```python
from build123d import *

# Parameters (mm, degrees)
F0_R     = 1.5
F0_R_2   = 10
F1_DEPTH = 3
F2_R     = 5


with BuildPart() as f1:
    # F0 (on Top) → F1 (new body)
    with BuildSketch(Plane.XY):
        with BuildLine():
            Line((67.5, 27.96), (27.96, 67.5))
            Line((27.96, 67.5), (7.0710678119, 46.6110678119))
            ThreePointArc((7.0710678119, 46.6110678119), (0, 43.6821356237), (-7.0710678119, 46.6110678119))
            Line((-7.0710678119, 46.6110678119), (-27.96, 67.5))
            Line((-27.96, 67.5), (-67.5, 27.96))
            Line((-67.5, 27.96), (-46.6110678119, 7.0710678119))
            ThreePointArc((-46.6110678119, 7.0710678119), (-43.6821356237, 0), (-46.6110678119, -7.0710678119))
            Line((-46.6110678119, -7.0710678119), (-67.5, -27.96))
            Line((-67.5, -27.96), (-27.96, -67.5))
            Line((-27.96, -67.5), (-7.0710678119, -46.6110678119))
            ThreePointArc((-7.0710678119, -46.6110678119), (0, -43.6821356237), (7.0710678119, -46.6110678119))
            Line((7.0710678119, -46.6110678119), (27.96, -67.5))
            Line((27.96, -67.5), (67.5, -27.96))
            Line((67.5, -27.96), (46.6110678119, -7.0710678119))
            ThreePointArc((46.6110678119, -7.0710678119), (43.6821356237, 0), (46.6110678119, 7.0710678119))
            Line((46.6110678119, 7.0710678119), (67.5, 27.96))
        make_face()
        with Locations((9.5, -35.5)):
            Circle(F0_R, mode=Mode.SUBTRACT)
        with Locations((35.3553390593, -35.3553390593)):
            Circle(F0_R_2, mode=Mode.SUBTRACT)
        with Locations((0, -21.9203102168)):
            Circle(F0_R, mode=Mode.SUBTRACT)
        with Locations((35.5, -9.5)):
            Circle(F0_R, mode=Mode.SUBTRACT)
        with Locations((-35.5, 9.5)):
            Circle(F0_R, mode=Mode.SUBTRACT)
        with Locations((-21.9203102168, 0)):
            Circle(F0_R, mode=Mode.SUBTRACT)
        with Locations((-35.3553390593, 35.3553390593)):
            Circle(F0_R_2, mode=Mode.SUBTRACT)
        with Locations((-9.5, 35.5)):
            Circle(F0_R, mode=Mode.SUBTRACT)
        with Locations((21.9203102168, 0)):
            Circle(F0_R, mode=Mode.SUBTRACT)
        with Locations((0, 21.9203102168)):
            Circle(F0_R, mode=Mode.SUBTRACT)
    extrude(amount=F1_DEPTH)

    # F2
    f2_edges = [f1.edges().sort_by_distance(p)[0] for p in [
        (27.96, -67.5, 1.5),
        (67.5, -27.96, 1.5),
        (67.5, 27.96, 1.5),
        (27.96, 67.5, 1.5),
        (-27.96, 67.5, 1.5),
        (-67.5, 27.96, 1.5),
        (-67.5, -27.96, 1.5),
        (-27.96, -67.5, 1.5),
    ]]
    fillet(f2_edges, radius=F2_R)


solid = f1.part
```
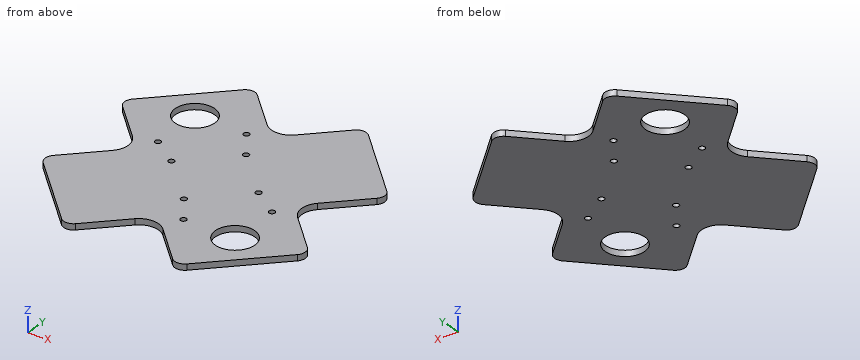
Build history of the part. All positions in model axes, mm. Coordinates: 2 decimals unless noted, no trailing zeros. Order: outer loops, then holes, each group sorted by start corner. A loop starts at its lowest first (then second) coordinate and runs counter-clockwise, first axis right, second up. Notation, with made-up numbers: M 57.25,-7 L 61.25,-7 A17 ccw 61.25,4 Z; hole C 10,45.25 d8. An arc over 180 degrees is marked long. One line per question, with ' | ' between items. Start each with the question number.
1. Flat gauge pins, fed straight in: P1, Ø4, axis at x = 21.92, y = 0, coming from the +Z side; P2, Ø1.5, axis at x = 9.5, z = 1.5, coming from the +Y side; P3, Ø1, axis at x = 4, z = 1.5, coming from the -Y side. Where does each tip first touch, or does it go through?
2. Cut at D-D (y = 29). Write the cut outline in (x, z), plus the area to 3 significant figures.
3. Wall check: line 1 along Y through (x, z) = (35.5, 0.7); line 2 along X through (y, z) = (-50, 1.6); line 3 along Y through (x, z) = (-39, 2). Give the ranges that are in metal, low to high. Write a range as [from, to].
4. Cut at A-A (y = 0). Write the cut outline in (x, z), plus the area to 3 significant figures.
5. Cut at B-B (x = 49). Write the cut outline in (y, z), plus the area to 3 significant figures.
The answers:
1) P1: stops at z = 3 | P2: stops at y = 49.79 | P3: stops at y = -44.75
2) outline: M -65.32,0 L -43.08,0 L -43.08,3 L -65.32,3 Z; M -27.63,0 L 65.32,0 L 65.32,3 L -27.63,3 Z | area: 346 mm2
3) line 1: y = [-59.96, -45.35], [-25.36, -11], [-8, 59.96] | line 2: x = [-45.46, -10.46], [10.46, 45.46] | line 3: y = [-56.46, 26.04], [44.67, 56.46]
4) outline: M -43.68,0 L -23.42,0 L -23.42,3 L -43.68,3 Z; M -20.42,0 L 20.42,0 L 20.42,3 L -20.42,3 Z; M 23.42,0 L 43.68,0 L 43.68,3 L 23.42,3 Z | area: 244 mm2
5) outline: M -46.46,0 L -9.46,0 L -9.46,3 L -46.46,3 Z; M 9.46,0 L 46.46,0 L 46.46,3 L 9.46,3 Z | area: 222 mm2
